```python
from build123d import *

# Parameters (mm, degrees)
F1_DEPTH    = 11
F2_W        = 20.4476909052
F2_H        = 25.2064025609
F3_DEPTH    = 15
F4_T1_DEPTH = 160.2446021291


# Not quite as in the source:
# - a fillet or chamfer that OpenCascade refuses, or shapes differently, is made with other operations: its cross-section is extruded or revolved along the edge and cut away or added


with BuildPart() as f1:
    # F0 (on Front) → F1 (new body)
    with BuildSketch(Plane.XZ):
        with BuildLine():
            Line((-10.2238454526, -37.989632494), (10.2238454526, -37.989632494))
            Line((10.2238454526, -37.989632494), (10.2238454526, 6.3570427475))
            Line((10.2238454526, 6.3570427475), (5.1648352034, 6.3570427475))
            ThreePointArc((5.1648352034, 6.3570427475), (0, 2.048837482), (-5.1648352034, 6.3570427475))
            Line((-5.1648352034, 6.3570427475), (-10.2238454526, 6.3570427475))
            Line((-10.2238454526, 6.3570427475), (-10.2238454526, -37.989632494))
        make_face()
    extrude(amount=F1_DEPTH)

    # F2 (on face) → F3 (join)
    with BuildSketch(Plane.XZ.offset(11)):
        with Locations((0, -25.3864312136)):
            Rectangle(F2_W, F2_H)
    extrude(amount=F3_DEPTH)

    # F4: fillet of radius 33.557568517 on 1 edges, made by hand

    # F4_s2 → F4_t1 (cut)
    with BuildSketch(Plane.YZ.offset(-80.1223010645)):
        with BuildLine():
            ThreePointArc((-26, -40.7426121779), (-22.0131710898, -24.8781309737), (-11, -12.7832299331))
            Line((-11, -12.7832299331), (-26, -12.7832299331))
            Line((-26, -12.7832299331), (-26, -40.7426121779))
        make_face()
    extrude(amount=F4_T1_DEPTH, mode=Mode.SUBTRACT)


solid = f1.part
```
Could you check a few things on this model? Use its own coordinates, in mm. Round coordinates to 2 decimals unless told otherwise and drop trailing zeros. Loops run counter-clockwise (first coordinate to the right, second up) from the corner with the lowest first, then second, coordinate; pieces in that order, holes last. Notation, with made-up numbers: M 25.25,-36.75 L 56.25,-36.75 A21 cw 56.25,-7.75 Z; hole C 82,34.25 d11. An arc over 180 degrees is marked long. Answer as CSV lines item,"result".
1) Imagine slicing it at B-B on y = -4. List the corners of the cut face in (x, z) for me.
From the geometry:
outline,"M -10.22,-37.99 L 10.22,-37.99 L 10.22,6.36 L 5.16,6.36 A5.25 cw -5.16,6.36 L -10.22,6.36 Z"
2) We'd pull the mould along X, two halves only. Please class faces 1 (the flat face through (-10.224, -10, -21)), 2 (the cylindrical face through (0.1, -5.42, 2.05)), 3 (the flat face through (0, -11, -3)): released by +X, released by -X, zero draft, split by the parting line, or undercut.
From the geometry:
face 1,"released by -X"
face 2,"undercut"
face 3,"zero draft"
3) Imagine slicing it at D-D on x = 4. List the corners of the cut face in (y, z) for me, and give its area (3 significant figures).
From the geometry:
outline,"M -25.89,-37.99 L 0,-37.99 L 0,3.9 L -11,3.9 L -11,-12.78 A33.56 ccw Z"
area,"715 mm^2"
4) Imagine slicing it at A-A on x = -6.5. List the corners of the cut face in (y, z) for me.
From the geometry:
outline,"M -25.89,-37.99 L 0,-37.99 L 0,6.36 L -11,6.36 L -11,-12.78 A33.56 ccw Z"
5) If I drill on probe 1 along Y at (x, z) = (-6, -4); probe 2 along Z at (x, y) = (3.25, -16.25); probe 3 along Y at (x, z) = (-8.5, -19), over which ranges is the centre line in solid material (lowest first)?
From the geometry:
probe 1,"-11 to 0"
probe 2,"-37.99 to -17.09"
probe 3,"-18 to 0"
6) Imagine slicing it at C-C on z = 0. List the corners of the cut face in (x, y) for me.
From the geometry:
outline,"M -10.22,-11 L 10.22,-11 L 10.22,0 L -10.22,0 Z"
7) For pin 1 Ø5.5 at (x, z) = (-4.5, -5) entering from -Y; pin 2 Ø6 at (x, y) = (-5.5, -13) entering from +Z; pin 3 Ø4 at (x, z) = (3.5, -24.5) entering from -Y; pin 4 Ø2 at (x, y) = (-0.5, -10) entering from +Z, each with a flat end and sliding along its axis, tell me the tip position at first contact or that it passes through.
From the geometry:
pin 1,"y = -11"
pin 2,"z = 6.36"
pin 3,"y = -22.83"
pin 4,"z = 2.27"
